from build123d import *

# Parameters (mm, degrees)
SKETCH1_W            = 196.85
SKETCH1_H            = 86.36
BOSS_EXTRUDE1_DEPTH  = 7.62
SKETCH7_W            = 63.5
SKETCH7_H            = 2.794
BOSS_EXTRUDE3_DEPTH  = 5.08
FILLET1_R            = 1.27
SKETCH6_R            = 2.3495
BOSS_EXTRUDE4_DEPTH  = 6.35
CUT_EXTRUDE3_DEPTH   = 4.064
SKETCH15_R           = 2.2479
CUT_EXTRUDE4_DEPTH   = 108.983537731
SKETCH17_R           = 3.3782
CUT_EXTRUDE5_DEPTH   = 108.74997645
SKETCH19_R           = 6.858
CUT_EXTRUDE6_DEPTH   = 4.064
SKETCH20_W           = 119.676272879
SKETCH20_H           = 31.665859335
CUT_EXTRUDE7_DEPTH   = 3.175
M3_CLEARANCE_HOLE1_D = 4.2
SKETCH26_R           = 3.05
CUT_EXTRUDE8_DEPTH   = 4
CHAMFER1_SIZE        = 7.62
CHAMFER1_SIZE2       = 6.35
FILLET5_R            = 1.27
FILLET6_R            = 4.318
FILLET7_R            = 1.778
FILLET8_R            = 0.762


with BuildPart() as part:
    # Sketch1 → Boss-Extrude1 (new body)
    with BuildSketch(Plane(origin=(0, 0, 0), x_dir=(1, 0, 0), z_dir=(0, 1, 0))):
        Rectangle(SKETCH1_W, SKETCH1_H)
    extrude(amount=BOSS_EXTRUDE1_DEPTH)

    # Sketch7 → Boss-Extrude3 (add)
    with BuildSketch(Plane(origin=(0, 7.62, 0), x_dir=(1, 0, 0), z_dir=(0, 1, 0))):
        with Locations((46.355, -41.783)):
            Rectangle(SKETCH7_W, SKETCH7_H)
    extrude(amount=BOSS_EXTRUDE3_DEPTH)

    # Fillet1
    fillet1_edges = [part.edges().sort_by_distance(p)[0] for p in [
        (14.605, 10.16, 40.386),
        (14.605, 10.16, 43.18),
        (78.105, 10.16, 43.18),
        (78.105, 10.16, 40.386),
    ]]
    fillet(fillet1_edges, radius=FILLET1_R)

    # Sketch6 → Boss-Extrude4 (add)
    with BuildSketch(Plane(origin=(0, 7.62, 0), x_dir=(1, 0, 0), z_dir=(0, 1, 0))):
        with Locations(Location((46.355, -22.606, 0), (0, 0, 270))):
            Circle(SKETCH6_R)
    extrude(amount=BOSS_EXTRUDE4_DEPTH)

    # Sketch14 → Cut-Extrude3 (cut)
    with BuildSketch(Plane(origin=(0, 7.62, 0), x_dir=(1, 0, 0), z_dir=(0, 1, 0))):
        Polygon((-53.213, 4.619379504), (-58.547, 4.619379504), (-61.214, 0), (-58.547, -4.619379504), (-53.213, -4.619379504), (-50.546, 0), align=None)
        Polygon((61.214, 0), (58.547, 4.619379504), (53.213, 4.619379504), (50.546, 0), (53.213, -4.619379504), (58.547, -4.619379504), align=None)
    extrude(amount=-CUT_EXTRUDE3_DEPTH, mode=Mode.SUBTRACT)

    # Sketch15 → Cut-Extrude4 (cut, through all)
    with BuildSketch(Plane(origin=(0, 3.556, 0), x_dir=(1, 0, 0), z_dir=(0, 1, 0))):
        with Locations(Location((-55.88, 0, 0), (0, 0, 270))):
            Circle(SKETCH15_R)
        with Locations(Location((55.88, 0, 0), (0, 0, 270))):
            Circle(SKETCH15_R)
    extrude(amount=-CUT_EXTRUDE4_DEPTH, mode=Mode.SUBTRACT)

    # Sketch17 → Cut-Extrude5 (cut, through all)
    with BuildSketch(Plane(origin=(0, 7.62, 0), x_dir=(1, 0, 0), z_dir=(0, 1, 0))):
        with Locations(Location((46.355, -8.636, 0), (0, 0, 270))):
            Circle(SKETCH17_R)
    extrude(amount=-CUT_EXTRUDE5_DEPTH, mode=Mode.SUBTRACT)

    # Sketch19 → Cut-Extrude6 (cut)
    with BuildSketch(Plane.XZ):
        with Locations(Location((46.355, 8.636, 0), (0, 0, 270))):
            Circle(SKETCH19_R)
    extrude(amount=-CUT_EXTRUDE6_DEPTH, mode=Mode.SUBTRACT)

    # Sketch20 → Cut-Extrude7 (cut)
    with BuildSketch(Plane.ZY.offset(98.425)):
        with Locations((11.670595095, 4.377895417)):
            Rectangle(SKETCH20_W, SKETCH20_H)
    extrude(amount=-CUT_EXTRUDE7_DEPTH, mode=Mode.SUBTRACT)

    # M3 Clearance Hole1 (through all)
    with Locations(Plane(origin=(0, 0, 0), x_dir=(-1, 0, 0), z_dir=(0, -1, 0))):
        with Locations((13.97, -19.177), (13.97, -0.889), (73.2282, -19.431), (62.23, 16.383324254)):
            Hole(M3_CLEARANCE_HOLE1_D / 2)

    # Sketch26 → Cut-Extrude8 (cut)
    with BuildSketch(Plane.XZ):
        with Locations(Location((-73.2282, 19.431, 0), (0, 0, 270))):
            Circle(SKETCH26_R)
        with Locations(Location((-62.23, -16.383324254, 0), (0, 0, 270))):
            Circle(SKETCH26_R)
        with Locations(Location((-13.97, 0.889, 0), (0, 0, 270))):
            Circle(SKETCH26_R)
        with Locations(Location((-13.97, 19.177, 0), (0, 0, 270))):
            Circle(SKETCH26_R)
    extrude(amount=-CUT_EXTRUDE8_DEPTH, mode=Mode.SUBTRACT)

    # Chamfer1
    chamfer1_edges = [part.edges().sort_by_distance(p)[0] for p in [
        (-95.25, 0, 0),
        (98.425, 0, 0),
    ]]
    chamfer1_side = [part.faces().sort_by_distance(p)[0] for p in [
        (1.4899049, 0, -0.118781761),
    ]]
    chamfer(chamfer1_edges, length=CHAMFER1_SIZE, length2=CHAMFER1_SIZE2, reference=chamfer1_side[0])

    # Fillet5
    # the kernel refuses this fillet: 1.27 mm, written as the material it takes off along each edge
    with BuildSketch(Plane(origin=(-95.25, 7.62, -46.355), x_dir=(1, 0, 0), z_dir=(0, 0, 1)), Plane(origin=(98.425, 7.62, -46.355), x_dir=(0, -1, 0), z_dir=(0, 0, 1))) as fillet5_piece_1:
        with BuildLine():
            CenterArc((FILLET5_R, -FILLET5_R), FILLET5_R, 90, 90)
            Line((0, -FILLET5_R), (0, 0))
            Line((0, 0), (FILLET5_R, 0))
        make_face()
    extrude(amount=92.71, mode=Mode.SUBTRACT)
    with BuildSketch(Plane(origin=(-95.25, 6.35, -44.667090454), x_dir=(0.7682212795973746, -0.6401843996644814, 0), z_dir=(0, 0, 1)), Plane(origin=(98.425, 6.35, -44.667090454), x_dir=(0, 1, 0), z_dir=(0, 0, 1))) as fillet5_piece_2:
        with BuildLine():
            CenterArc((FILLET5_R * 0.468374945984, FILLET5_R), FILLET5_R, 219.805571092, 50.194428908)
            Line((-FILLET5_R * 0.299846333613, FILLET5_R * 0.359815600336), (0, 0))
            Line((0, 0), (FILLET5_R * 0.468374945984, 0))
        make_face()
    extrude(amount=89.334180907, mode=Mode.SUBTRACT)

    # Fillet6
    fillet6_edges = [part.edges().sort_by_distance(p)[0] for p in [
        (90.805, 0, 0),
        (-87.63, 0, 0),
    ]]
    fillet(fillet6_edges, radius=FILLET6_R)

    # Fillet7
    # the kernel refuses this fillet: 1.778 mm, written as the material it takes off along each edge
    with BuildSketch(Plane(origin=(-88.830984618, 1.000820515, 43.18), x_dir=(0.6401843996644796, 0.768221279597376, 0), z_dir=(-0.7682212795973761, 0.6401843996644797, 0)), Plane(origin=(-88.830984618, 1.000820515, -43.18), x_dir=(0, 0, 1), z_dir=(-0.7682212795973761, 0.6401843996644797, 0))) as fillet7_piece_1:
        with BuildLine():
            CenterArc((FILLET7_R, FILLET7_R), FILLET7_R, 180, 90)
            Line((0, FILLET7_R), (0, 0))
            Line((0, 0), (FILLET7_R, 0))
        make_face()
    extrude(amount=12.205849287, mode=Mode.SUBTRACT)
    with BuildSketch(Plane(origin=(-86.06666838, 4.318, 43.18), x_dir=(0, -1, 0), z_dir=(1, 0, 0))) as fillet7_piece_2:
        with BuildLine():
            CenterArc((4.318 - FILLET7_R, FILLET7_R), FILLET7_R, 270, 90)
            Line((4.318, FILLET7_R), (4.318, 0))
            Line((4.318, 0), (4.318 - FILLET7_R, 0))
        make_face()
    revolve(axis=Axis((-86.06666838, 4.318, 43.18), (0, 0, -1)), revolution_arc=39.805571092, mode=Mode.SUBTRACT)
    with BuildSketch(Plane(origin=(92.005984618, 1.000820515, 43.18), x_dir=(-0.6401843996644796, 0.768221279597376, 0), z_dir=(0.7682212795973761, 0.6401843996644797, 0)), Plane(origin=(92.005984618, 1.000820515, -43.18), x_dir=(0, 0, 1), z_dir=(0.7682212795973761, 0.6401843996644797, 0))) as fillet7_piece_3:
        with BuildLine():
            CenterArc((FILLET7_R, -FILLET7_R), FILLET7_R, 90, 90)
            Line((0, -FILLET7_R), (0, 0))
            Line((0, 0), (FILLET7_R, 0))
        make_face()
    extrude(amount=12.205849287, mode=Mode.SUBTRACT)
    with BuildSketch(Plane(origin=(89.24166838, 4.318, 43.18), x_dir=(0, -1, 0), z_dir=(-1, 0, 0))) as fillet7_piece_4:
        with BuildLine():
            CenterArc((4.318 - FILLET7_R, -FILLET7_R), FILLET7_R, 0, 90)
            Line((4.318, -FILLET7_R), (4.318, 0))
            Line((4.318, 0), (4.318 - FILLET7_R, 0))
        make_face()
    revolve(axis=Axis((89.24166838, 4.318, 43.18), (0, 0, 1)), revolution_arc=39.805571092, mode=Mode.SUBTRACT)
    with BuildSketch(Plane(origin=(89.24166838, 0, 43.18), x_dir=(0, 1, 0), z_dir=(-1, 0, 0))) as fillet7_piece_5:
        with BuildLine():
            CenterArc((FILLET7_R, FILLET7_R), FILLET7_R, 180, 90)
            Line((0, FILLET7_R), (0, 0))
            Line((0, 0), (FILLET7_R, 0))
        make_face()
    extrude(amount=175.30833676, mode=Mode.SUBTRACT)
    with BuildSketch(Plane(origin=(89.24166838, 4.318, -43.18), x_dir=(0, -1, 0), z_dir=(-1, 0, 0))) as fillet7_piece_6:
        with BuildLine():
            CenterArc((4.318 - FILLET7_R, FILLET7_R), FILLET7_R, 270, 90)
            Line((4.318 - FILLET7_R, 0), (4.318, 0))
            Line((4.318, 0), (4.318, FILLET7_R))
        make_face()
    revolve(axis=Axis((89.24166838, 4.318, -43.18), (0, 0, 1)), revolution_arc=39.805571092, mode=Mode.SUBTRACT)
    with BuildSketch(Plane(origin=(-86.06666838, 4.318, -43.18), x_dir=(0, -1, 0), z_dir=(1, 0, 0))) as fillet7_piece_7:
        with BuildLine():
            CenterArc((4.318 - FILLET7_R, -FILLET7_R), FILLET7_R, 0, 90)
            Line((4.318 - FILLET7_R, 0), (4.318, 0))
            Line((4.318, 0), (4.318, -FILLET7_R))
        make_face()
    revolve(axis=Axis((-86.06666838, 4.318, -43.18), (0, 0, -1)), revolution_arc=39.805571092, mode=Mode.SUBTRACT)
    with BuildSketch(Plane(origin=(-86.06666838, 0, -43.18), x_dir=(0, 0, 1), z_dir=(1, 0, 0))) as fillet7_piece_8:
        with BuildLine():
            CenterArc((FILLET7_R, -FILLET7_R), FILLET7_R, 90, 90)
            Line((0, -FILLET7_R), (0, 0))
            Line((0, 0), (FILLET7_R, 0))
        make_face()
    extrude(amount=175.30833676, mode=Mode.SUBTRACT)

    # Fillet8
    fillet8_edges = [part.edges().sort_by_distance(p)[0] for p in [
        (14.605, 12.7, 41.783),
        (46.355, 12.7, 40.386),
        (46.355, 12.7, 43.18),
        (78.105, 12.7, 41.783),
        (77.733025612, 12.7, 42.808025612),
        (77.733025612, 12.7, 40.757974388),
        (14.976974388, 12.7, 42.808025612),
        (14.976974388, 12.7, 40.757974388),
        (46.355, 13.97, 20.2565),
    ]]
    fillet(fillet8_edges, radius=FILLET8_R)


solid = part.part
Source: CAD feature listing. Evaluate the final solid. Frame: model axes, mm. A direction names the side the tool comes from. Coordinates: 2 decimals unless noted, no trailing zeros. Write each loop counter-clockwise with the first axis right and the second up, starting at its lowest first coordinate (ties: lowest second). Pieces come first, ordered by that corner, then holes. Notation, with made-up numbers: M -14.5,-8.75 L 4.5,-8.75 A23 ccw 4.5,27.25 Z; hole C 83.5,-8 d8. An arc over 180 degrees is marked long. Use a Markdown table: item, result.
1) Mould query, pull axis X, two halves, no side actions, for faces 1 (the flat face through (45, 4.064, 12)), 2 (the flat face through (-59.862, 5.616, -2.342)), 3 (the flat face through (-91.854, 3.52, -0.58)), 4 (the cylindrical face through (44.06, 10.37, 22.1)). Classes: pulls with the +X half, pulls with the -X half, needs draft (parallel to the pull), parting line crosses it, or undercut.
Conclusion:
| item | result |
|---|---|
| face 1 | undercut |
| face 2 | undercut |
| face 3 | pulls with the -X half |
| face 4 | parting line crosses it |
2) Section B-B, the plane x = 55.88. Output: boundary loops of the cut face in (y, z), then the cut area to 3 significant figures.
Conclusion:
| item | result |
|---|---|
| outline | M 0,-41.4 A1.78 ccw 1.78,-43.18 L 7.62,-43.18 L 7.62,-4.62 L 3.56,-4.62 L 3.56,-2.25 L 0,-2.25 Z; M 0,2.25 L 3.56,2.25 L 3.56,4.62 L 7.62,4.62 L 7.62,40.39 L 11.94,40.39 A0.76 ccw 12.7,41.15 L 12.7,42.42 A0.76 ccw 11.94,43.18 L 1.78,43.18 A1.78 ccw 0,41.4 Z |
| area | 617 mm^2 |
3) Reachability of faces 5 (the flat face through (-73, 4, 17)), 6 (the flat face through (58.2, 3.556, -1.1)), 7 (the cylindrical face through (95, 4.1, -42.6)) from +Z, -Z, +X, -X, +Y, -Y: full face, straight path, thin tool, end or side. Return the list, or none.
Conclusion:
| item | result |
|---|---|
| face 5 | -Y |
| face 6 | +Y |
| face 7 | -Z, +X, -Y |
4) First-contact query: pin 1 Ø4 at (y, z) = (4, 17) entering from -X; pin 2 Ø8 at (y, z) = (8, -28) entering from -X; pin 3 Ø3 at (x, z) = (-53.5, -2) entering from +Y. Flat tips, straight axial feed; report the tip coordinate or a pass-through.
Conclusion:
| item | result |
|---|---|
| pin 1 | stops at x = -94.83 |
| pin 2 | stops at x = -95.21 |
| pin 3 | stops at y = 3.56 |
5) Ray query, L1, parallel to X at y = 2.5, z = 0 (3 decimals); L2, parallel to Y at x = 35, z = 26.5; L3, parallel to X at y = 0.5, z = 18. Return the intervals inside material, ascending.
Conclusion:
| item | result |
|---|---|
| L1 | x = -90.63 to -58.128, -53.632 to -16.888, -11.052 to 53.632, 58.128 to 93.805 |
| L2 | y = 0 to 7.62 |
| L3 | x = -88.08 to -75.92, -70.53 to -16.78, -11.16 to 91.26 |
6) Section A-A, the plane x = -13.97. Output: boundary loops of the cut face in (y, z).
Conclusion:
| item | result |
|---|---|
| outline | M 0,-41.4 A1.78 ccw 1.78,-43.18 L 7.62,-43.18 L 7.62,-1.21 L 4,-1.21 L 4,-2.16 L 0,-2.16 Z; M 0,3.94 L 4,3.94 L 4,2.99 L 7.62,2.99 L 7.62,17.08 L 4,17.08 L 4,16.13 L 0,16.13 Z; M 0,22.23 L 4,22.23 L 4,21.28 L 7.62,21.28 L 7.62,43.18 L 1.78,43.18 A1.78 ccw 0,41.4 Z |
7) Section D-D, the plane x = 26.5. Output: boundary loops of the cut face in (y, z), then the cut area to 3 significant figures.
Conclusion:
| item | result |
|---|---|
| outline | M 0,-41.4 A1.78 ccw 1.78,-43.18 L 7.62,-43.18 L 7.62,40.39 L 11.94,40.39 A0.76 ccw 12.7,41.15 L 12.7,42.42 A0.76 ccw 11.94,43.18 L 1.78,43.18 A1.78 ccw 0,41.4 Z |
| area | 671 mm^2 |
8) Section C-C, the plane z = 9. Output: boundary loops of the cut face in (x, y) (3 decimals).
Conclusion:
| item | result |
|---|---|
| outline | M -95.215,6.647 A1.27 ccw -94.793,5.969 L -88.831,1.001 A4.318 ccw -86.067,0 L 39.507,0 L 39.507,4.064 L 42.996,4.064 L 42.996,7.62 L -93.98,7.62 A1.27 ccw Z; M 49.714,4.064 L 53.203,4.064 L 53.203,0 L 89.242,0 A4.318 ccw 92.006,1.001 L 97.968,5.969 A1.27 ccw 98.39,6.647 A1.27 ccw 97.155,7.62 L 49.714,7.62 Z |
